from build123d import *

# Parameters (mm, degrees)
SKETCH2_W           = 30
SKETCH2_H           = 27
BOSS_EXTRUDE1_DEPTH = 20
SKETCH6_W           = 4
SKETCH6_H           = 27
CUT_EXTRUDE4_DEPTH  = 26
SKETCH9_W           = 6
SKETCH9_H           = 19
CUT_EXTRUDE5_DEPTH  = 20
SKETCH11_R          = 5
CUT_EXTRUDE8_DEPTH  = 0.5
SKETCH12_W          = 2.75
SKETCH12_H          = 12
CUT_EXTRUDE12_DEPTH = 17.5
SKETCH15_R          = 4.5
CUT_EXTRUDE13_DEPTH = 10


with BuildPart() as part:
    # Sketch2 → Boss-Extrude1 (new body)
    with BuildSketch(Plane(origin=(0, 0, 0), x_dir=(0, 0, -1), z_dir=(1, 0, 0))):
        with Locations((15, 13.5)):
            Rectangle(SKETCH2_W, SKETCH2_H)
    extrude(amount=BOSS_EXTRUDE1_DEPTH)

    # Sketch6 → Cut-Extrude4 (cut)
    with BuildSketch(Plane(origin=(2.296116437, 27, -0.293484995), x_dir=(1, 0, 0), z_dir=(0, 1, 0))):
        with Locations((13.365844825, 14.706515005)):
            Rectangle(SKETCH6_W, SKETCH6_H)
    extrude(amount=-CUT_EXTRUDE4_DEPTH, mode=Mode.SUBTRACT)

    # Sketch9 → Cut-Extrude5 (cut)
    with BuildSketch(Plane(origin=(0, 27, 0), x_dir=(1, 0, 0), z_dir=(0, 1, 0))):
        with Locations((10.661961261, 15)):
            Rectangle(SKETCH9_W, SKETCH9_H)
    extrude(amount=-CUT_EXTRUDE5_DEPTH, mode=Mode.SUBTRACT)

    # Sketch11 → Cut-Extrude8 (cut)
    with BuildSketch(Plane.ZY):
        with Locations((-15.1, 13.5)):
            Circle(SKETCH11_R)
    extrude(amount=-CUT_EXTRUDE8_DEPTH, mode=Mode.SUBTRACT)

    # Sketch12 → Cut-Extrude12 (cut)
    with BuildSketch(Plane(origin=(0, 27, 0), x_dir=(1, 0, 0), z_dir=(0, 1, 0))):
        with Locations((5.286961261, 15)):
            Rectangle(SKETCH12_W, SKETCH12_H)
    extrude(amount=-CUT_EXTRUDE12_DEPTH, mode=Mode.SUBTRACT)

    # Sketch15 → Cut-Extrude13 (cut)
    with BuildSketch(Plane.ZY.offset(-0.5)):
        with Locations((-15.04, 13.5)):
            Circle(SKETCH15_R)
    extrude(amount=-CUT_EXTRUDE13_DEPTH, mode=Mode.SUBTRACT)


solid = part.part
The model under review builds one solid part; all positions refer to its coordinate system, in mm. A direction names the side the tool comes from. Coordinates: 2 decimals unless noted, no trailing zeros. Write each loop counter-clockwise with the first axis right and the second up, starting at its lowest first coordinate (ties: lowest second). Pieces come first, ordered by that corner, then holes. Notation, with made-up numbers: (59.25, -38.5) - (102.25, -38.5) arc R23 cw to (102.25, -24.5) - close; hole circle Ø4 at (26.25, 18.25). An arc over 180 degrees is marked (long way). Answer as a JSON object with one key per item and string values. Group by question number.
1. Clearance check with flat-ended pins moving along their axes: pin 1 Ø1.5 at (x, z) = (16, -10) entering from +Y; pin 2 Ø2 at (x, z) = (5, -12) entering from +Y; pin 3 Ø6 at (y, z) = (13.5, -15.1) entering from -X. State where each tip first meets the part, or that it passes through.
2. Machinability: for faces 4 (the face through (0, 8, -15)), 5 (the face through (5, 9.5, -19)), 6 (the face through (0.246, 11.585, -10.481)), which of the approach directions +Z, -Z, +X, -X, +Y, -Y give a long, thin tool a straight path to every point of the face, cutting with its end or side? Answer none if there is none.
3. Add section D-D (z = -15.1). Give the boundary of the cut face in (x, y).
4. Add section C-C (x = 11.75). Give the boundary of the cut face in (y, z).
5. Add section B-B (z = -7). Give the boundary of the cut face in (x, y).
6. Mouldability with a two-part tool opening along Y and no side actions: class faces 1 (the face through (10, 0, -15)), 2 (the face through (0.5, 11, -19)), 3 (the face through (20, 14, -15)) as pulls with the +Y half, pulls with the -Y half, needs draft (parallel to the pull), parting line crosses it, or undercut.
7. To check wall thickness, follow probe 1 along X at (y, z) = (23.5, -13.75); probe 2 along X at (y, z) = (21.75, -3.75); probe 3 along Z at (x, y) = (7, 13.25). State the ranges of each line that lie inside material, in increasing order.
8. Add section A-A (y = 13.5). Give the boundary of the cut face in (x, z).
Findings:
{
 "1": {"pin 1": "y = 1", "pin 2": "y = 9.5", "pin 3": "x = 17.66"},
 "2": {"face 4": "+Z, -Z, -X, +Y, -Y", "face 5": "+Y", "face 6": "-X"},
 "3": {"outline": "(0, 0) - (20, 0) - (20, 27) - (17.66, 27) - (17.66, 1) - (13.66, 1) - (13.66, 7) - (7.66, 7) - (7.66, 9) - (0.5, 9) - (0.5, 8.5) - (0, 8.5) - close; (0, 18.5) - (0.5, 18.5) - (0.5, 18) - (3.91, 18) - (3.91, 27) - (0, 27) - close; (6.66, 18) - (7.66, 18) - (7.66, 27) - (6.66, 27) - close"},
 "4": {"outline": "(0, -30) - (27, -30) - (27, -24.5) - (7, -24.5) - (7, -5.5) - (27, -5.5) - (27, 0) - (0, 0) - close"},
 "5": {"outline": "(0, 0) - (20, 0) - (20, 27) - (17.66, 27) - (17.66, 1) - (13.66, 1) - (13.66, 7) - (7.66, 7) - (7.66, 27) - (0, 27) - close"},
 "6": {"face 1": "pulls with the -Y half", "face 2": "undercut", "face 3": "needs draft"},
 "7": {"probe 1": "0 to 3.91, 6.66 to 7.66, 17.66 to 20", "probe 2": "0 to 13.66, 17.66 to 20", "probe 3": "-30 to -19.53, -10.55 to 0"},
 "8": {"outline": "(0, -30) - (20, -30) - (20, 0) - (0, 0) - (0, -10.1) - (0.5, -10.1) - (0.5, -10.54) - (3.91, -10.54) - (3.91, -9) - (6.66, -9) - (6.66, -10.54) - (7.66, -10.54) - (7.66, -5.5) - (13.66, -5.5) - (13.66, -1.5) - (17.66, -1.5) - (17.66, -28.5) - (13.66, -28.5) - (13.66, -24.5) - (7.66, -24.5) - (7.66, -19.54) - (6.66, -19.54) - (6.66, -21) - (3.91, -21) - (3.91, -19.54) - (0.5, -19.54) - (0.5, -20.1) - (0, -20.1) - close"}
}
